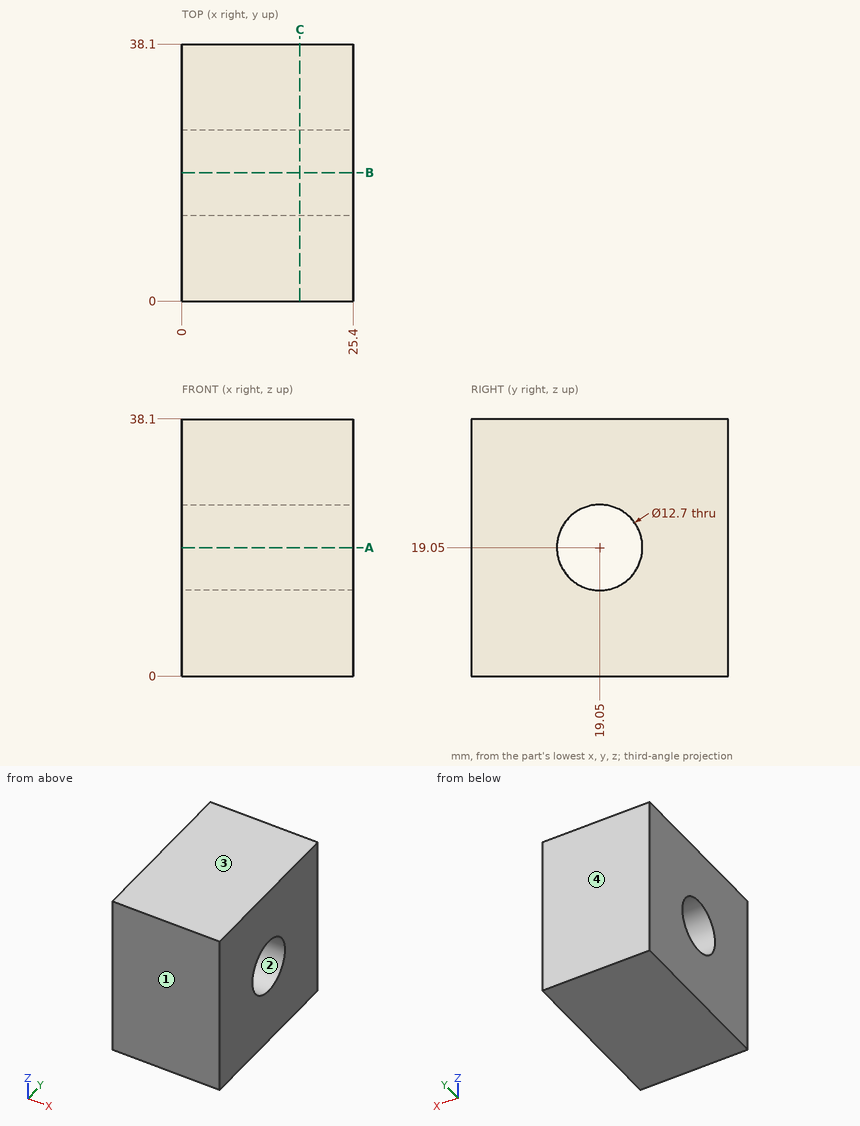
The figure shows three views and two pictorial views of one solid part (mm, origin at its lowest corner). Answer the questions. Round coordinates to 2 decimals unless told otherwise and drop trailing zeros. Order: outer loops, then holes, each group sorted by start corner. A loop starts at its lowest first (then second) coordinate and runs counter-clockwise, first axis right, second up.
Q1. A cutting plane is placed at A-A, the plane z = 19.05. Determine the outline of the cut face in (x, y).
Solution:
outline: (0, 0) - (25.4, 0) - (25.4, 12.7) - (0, 12.7) - close; (0, 25.4) - (25.4, 25.4) - (25.4, 38.1) - (0, 38.1) - close
Q2. Find the intervals of material crossed by line 1 along Y through (x, z) = (12, 19.05); line 2 along Z through (x, y) = (12, 21); line 3 along Z through (x, y) = (9, 24.5), in increasing order.
Solution:
line 1: y = 0 to 12.7, 25.4 to 38.1
line 2: z = 0 to 13.01, 25.09 to 38.1
line 3: z = 0 to 15.79, 22.31 to 38.1
Q3. Given pin 1 Ø6 at (x, y) = (16.5, 12) entering from -Z, flat-ended and moving along its own axis, determine where the tip first touches the part or whether it passes through.
Solution:
pin 1: stops at z = 0
Q4. The mould has two halves that part along Y. Classify the marked faces 1, 2, 3 and 4: pulls with the +Y half, pulls with the -Y half, needs draft (parallel to the pull), parting line crosses it, or undercut.
Solution:
face 1: pulls with the -Y half
face 2: undercut
face 3: needs draft
face 4: pulls with the +Y half
Q5. A cutting plane is placed at C-C, the plane x = 17.5. Determine the outline of the cut face in (y, z).
Solution:
outline: (0, 0) - (38.1, 0) - (38.1, 38.1) - (0, 38.1) - close; hole circle Ø12.7 at (19.05, 19.05)
